Verification items for the finished model (mm, model axes). Give positions to 0.01 mm unless a question says otherwise; leave off trailing zeros. Write each loop counter-clockwise with the first axis right and the second up, starting at its lowest first coordinate (ties: lowest second). Pieces come first, ordered by that corner, then holes. Notation, with made-up numbers: (-33, -30) -> (-20, -30) arc R34 ccw to (-20, 3) -> close; hole circle Ø9 at (-21, 58.25). An arc over 180 degrees is marked (long way). Use one line per item in the form item = value. Start each with the question number.
(1) Depth check by flat-ended pin: pin 1 Ø2.5 at (x, z) = (105.92, 7.74) entering from +Y. Enter the tip coordinate at first touch or a pass-through.
(2) Section check A-A, the plane y = -4.25. Record the cut outline in (x, z).
(3) Scan lines: L1, parallel to Z at x = 109, y = -5; L2, parallel to Y at x = 215.5, z = -11. Record each from-to range of solid material in increasing order.
(4) Section check B-B, the plane z = 0.5. Record the cut outline in (x, y).
(5) Section check C-C, the plane x = 349.5. Record the cut outline in (y, z), plus the area to 3 significant figures.
from build123d import *

# Parameters (mm, degrees)
SKETCH_1_W          = 40
SKETCH_1_H          = 20
EXTRUDE_1_DEPTH     = 391
SHELL_1_T           = -1
SKETCH_2_R          = 1.5
CUT_EXTRUDE_1_DEPTH = 48
SKETCH_3_R          = 1.25
CUT_EXTRUDE_2_DEPTH = 37


with BuildPart() as part:
    # 草图1 → 凸台-拉伸1 (new body)
    with BuildSketch(Plane(origin=(0, 0, 0), x_dir=(0, 0, -1), z_dir=(1, 0, 0))):
        Rectangle(SKETCH_1_W, SKETCH_1_H)
    extrude(amount=EXTRUDE_1_DEPTH)

    # 抽壳1
    shell_1_openings = [part.faces().sort_by_distance(p)[0] for p in [
        (391, 0, 0),
        (0, 0, 0),
    ]]
    offset(amount=SHELL_1_T, openings=shell_1_openings, kind=Kind.INTERSECTION)

    # 草图2 → 切除-拉伸1 (cut)
    with BuildSketch(Plane(origin=(0, 10, 0), x_dir=(1, 0, 0), z_dir=(0, 1, 0))):
        with Locations(Location((15.921137183, 7.495400719, 0), (0, 0, 270))):
            Circle(SKETCH_2_R)
        with Locations(Location((45.921137183, 7.495400719, 0), (0, 0, 270))):
            Circle(SKETCH_2_R)
        with Locations(Location((75.921137183, 7.495400719, 0), (0, 0, 270))):
            Circle(SKETCH_2_R)
        with Locations(Location((105.921137183, 7.495400719, 0), (0, 0, 270))):
            Circle(SKETCH_2_R)
        with Locations(Location((135.921137183, 7.495400719, 0), (0, 0, 270))):
            Circle(SKETCH_2_R)
        with Locations(Location((15.921137183, -7.735756338, 0), (0, 0, 270))):
            Circle(SKETCH_2_R)
        with Locations(Location((45.921137183, -7.735756338, 0), (0, 0, 270))):
            Circle(SKETCH_2_R)
        with Locations(Location((75.921137183, -7.735756338, 0), (0, 0, 270))):
            Circle(SKETCH_2_R)
        with Locations(Location((105.921137183, -7.735756338, 0), (0, 0, 270))):
            Circle(SKETCH_2_R)
        with Locations(Location((135.921137183, -7.735756338, 0), (0, 0, 270))):
            Circle(SKETCH_2_R)
    extrude(amount=-CUT_EXTRUDE_1_DEPTH, mode=Mode.SUBTRACT)

    # 草图3 → 切除-拉伸2 (cut)
    with BuildSketch(Plane.XZ.offset(10)):
        with Locations(Location((354.561034917, -13.835401739, 0), (0, 0, 270))):
            Circle(SKETCH_3_R)
        with Locations(Location((381.426907587, -13.361180576, 0), (0, 0, 270))):
            Circle(SKETCH_3_R)
        with Locations(Location((380.952686425, 13.504692093, 0), (0, 0, 270))):
            Circle(SKETCH_3_R)
        with Locations(Location((354.086813755, 13.030470931, 0), (0, 0, 270))):
            Circle(SKETCH_3_R)
    extrude(amount=-CUT_EXTRUDE_2_DEPTH, mode=Mode.SUBTRACT)


solid = part.part
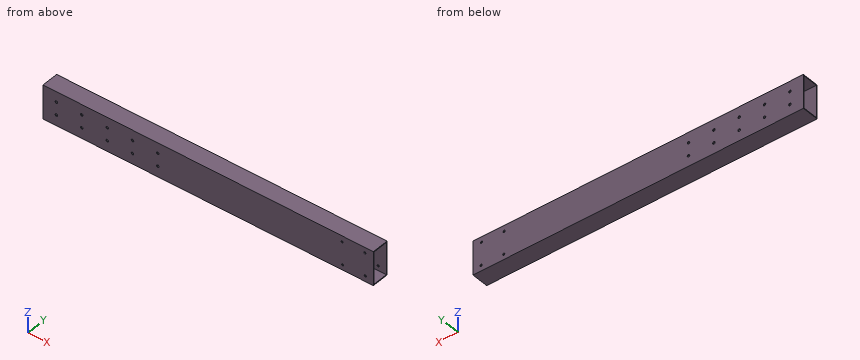
Completed:
q1.pin_1 = through
q2.outline = (0, -20) -> (391, -20) -> (391, -19) -> (0, -19) -> close; (0, 19) -> (391, 19) -> (391, 20) -> (0, 20) -> close
q3.L1 = -20 to -19, 19 to 20
q3.L2 = -10 to -9, 9 to 10
q4.outline = (0, -10) -> (391, -10) -> (391, -9) -> (0, -9) -> close; (0, 9) -> (391, 9) -> (391, 10) -> (0, 10) -> close
q5.outline = (-10, -20) -> (10, -20) -> (10, 20) -> (-10, 20) -> close; hole (-9, -19) -> (9, -19) -> (9, 19) -> (-9, 19) -> close
q5.area = 116 mm²
